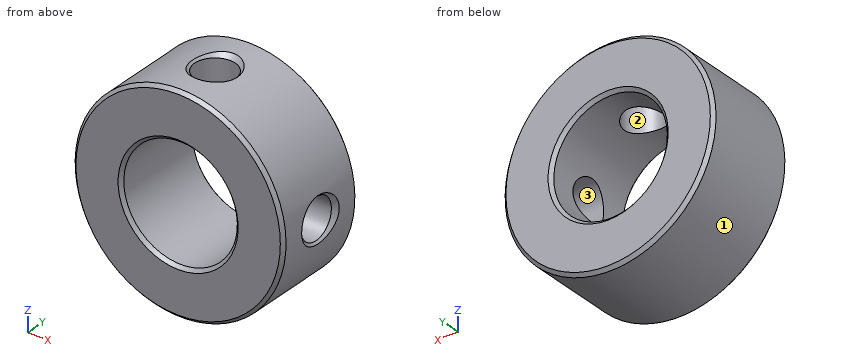
```python
from build123d import *

# Parameters (mm, degrees)
PROFILES_R        = 6.5
PROFILES_R_2      = 3.5
PROFILE_DEPTH     = 3
CIRPATTERN1_COUNT = 2
CIRPATTERN1_ANGLE = 90
OUTERC_SIZE       = 0.2
INNERC_SIZE       = 0.2


# Read off the part's stored shape, not the designer's step:  Tapped Hole1
with BuildPart() as part:
    # ProfileS → Profile (new, symmetric)
    with BuildSketch(Plane(origin=(0, 0, 0), x_dir=(1, 0, 0), z_dir=(0, 1, 0))):
        with Locations(Location((0, 0, 0), (0, 0, 270))):
            Circle(PROFILES_R)
        with Locations(Location((0, 0, 0), (0, 0, 270))):
            Circle(PROFILES_R_2, mode=Mode.SUBTRACT)
    extrude(amount=PROFILE_DEPTH, both=True)

    # Tapped Hole1 outline → Tapped Hole1 (revolve, cut)
    with BuildSketch(Plane.XZ):
        Polygon((1.525000359, 6.500000359), (0, 6.500000359), (0, 3.269069771), (1.25, 3.269069771), (1.25, 6.225), align=None)
    tapped_hole1 = revolve(axis=Axis((0, 0, 0), (0, 0, 1)), mode=Mode.SUBTRACT)

    # CirPattern1: Tapped Hole1 ×2 about axis
    cirpattern1_axis = Axis((0, 3, 0), (0, 1, 0))
    for i in range(1, CIRPATTERN1_COUNT):
        add(tapped_hole1.rotate(cirpattern1_axis, i * CIRPATTERN1_ANGLE / (CIRPATTERN1_COUNT - 1)), mode=Mode.SUBTRACT)

    # OuterC
    outerc_edges = [part.edges().sort_by_distance(p)[0] for p in [
        (0, -3, -6.5),
        (0, 3, -6.5),
    ]]
    chamfer(outerc_edges, length=OUTERC_SIZE)

    # InnerC
    innerc_edges = [part.edges().sort_by_distance(p)[0] for p in [
        (0, -3, -3.5),
        (0, 3, -3.5),
    ]]
    chamfer(innerc_edges, length=INNERC_SIZE)


solid = part.part
```
Input: part model. Units: mm. Frame: model coordinates. Face numbers are marked on the shaded views. Give positions to 0.01 mm unless a question says otherwise; leave off trailing zeros. Write each loop counter-clockwise with the first axis right and the second up, starting at its lowest first coordinate (ties: lowest second). Pieces come first, ordered by that corner, then holes. Notation, with made-up numbers: (32, -10.75) - (76, -10.75) arc R18 ccw to (76, 13.25) - close; hole circle Ø1 at (19, 85.25). An arc over 180 degrees is marked (long way). Write item = value, one per line. Start each with the question number.
1. Section query A-A, the plane x = 0. Output: boundary loops of the cut face in (y, z) (3 decimals), then the cut area to 3 significant figures.
2. First-contact query: pin 1 Ø6.5 at (x, z) = (0, 0) entering from +Y; pin 2 Ø3 at (x, y) = (4, -0.5) entering from +Z. Flat tips, straight axial feed; report the tip coordinate or a pass-through.
3. Mould query, pull axis Z, two halves, no side actions, for the marked faces 1, 2 and 3. Classes: released by +Z, released by -Z, zero draft, split by the parting line, or undercut.
4. Section query B-B, the plane y = 0. Output: boundary loops of the cut face in (x, z) (3 decimals), then the cut area to 3 significant figures.
5. Ray query, L1, parallel to Y at x = 0, z = 5; L2, parallel to X at y = 0.45, z = 0; L3, parallel to X at y = 1.8, z = 0.75. Return the intervals inside material, ascending.
6. Section query C-C, the plane y = -2.35. Output: boundary loops of the cut face in (x, z).
Check sheet entries:
q1.outline = (-3, -6.3) - (-2.8, -6.5) - (2.8, -6.5) - (3, -6.3) - (3, -3.7) - (2.8, -3.5) - (-2.8, -3.5) - (-3, -3.7) - close; (-3, 3.7) - (-2.8, 3.5) - (-1.25, 3.5) - (-1.25, 6.225) - (-1.525, 6.5) - (-2.8, 6.5) - (-3, 6.3) - close; (1.25, 3.5) - (2.8, 3.5) - (3, 3.7) - (3, 6.3) - (2.8, 6.5) - (1.525, 6.5) - (1.25, 6.225) - close
q1.area = 28.3 mm2
q2.pin_1 = through
q2.pin_2 = 6
q3.face_1 = split by the parting line
q3.face_2 = zero draft
q3.face_3 = undercut
q4.outline = (-1.377, 6.352) arc R6.5 ccw (long way) to (6.352, -1.377) - (6.225, -1.25) - (3.269, -1.25) arc R3.5 cw (long way) to (-1.25, 3.269) - (-1.25, 6.225) - close; (1.25, 3.269) arc R3.5 cw to (3.269, 1.25) - (6.225, 1.25) - (6.352, 1.377) arc R6.5 ccw to (1.377, 6.352) - (1.25, 6.225) - close
q4.area = 79.0 mm2
q5.L1 = -3 to -1.25, 1.25 to 3
q5.L2 = -6.5 to -3.5
q5.L3 = -6.46 to -3.42, 3.42 to 6.46
q6.outline = circle Ø13 at (0, 0); hole circle Ø7 at (0, 0)
